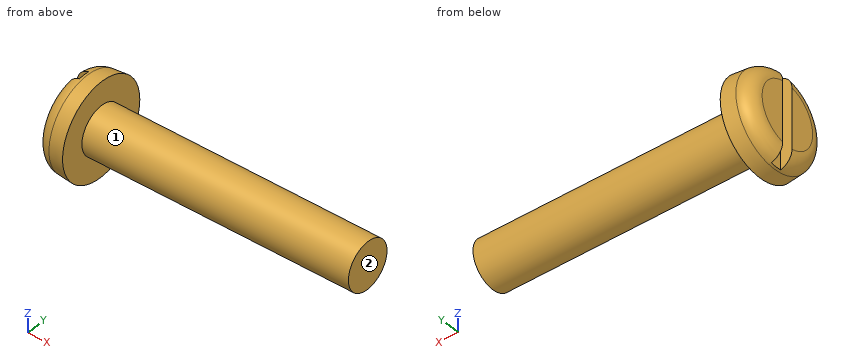
from build123d import *

# Parameters (mm, degrees)
FILLET2_R  = 0.8
SKETCH2_W  = 5
SKETCH2_H  = 0.6
SLOT_DEPTH = 0.6


with BuildPart() as part:
    # BodySke → Base-Revolve (revolve)
    with BuildSketch(Plane.XY):
        Polygon((1.5, 1.25), (1.5, 2.5), (0, 2.368767005), (0, 0), (15.5, 0), (15.5, 1.25), align=None)
    revolve(axis=Axis((-25.4, 0, 0), (1, 0, 0)))

    # Fillet2
    fillet2_edges = [part.edges().sort_by_distance(p)[0] for p in [
        (0, -2.368767005, 0),
    ]]
    fillet(fillet2_edges, radius=FILLET2_R)

    # Sketch2 → Slot (cut)
    with BuildSketch(Plane(origin=(0, 0, 0), x_dir=(0, 0, -1), z_dir=(1, 0, 0))):
        Rectangle(SKETCH2_W, SKETCH2_H)
    extrude(amount=SLOT_DEPTH, mode=Mode.SUBTRACT)


solid = part.part
Read the model definition and answer for the solid it produces. Units are mm, in the model's axes. Face numbers are marked on the shaded views. A direction names the side the tool comes from. Round coordinates to 2 decimals unless told otherwise and drop trailing zeros. Write each loop counter-clockwise with the first axis right and the second up, starting at its lowest first coordinate (ties: lowest second). Pieces come first, ordered by that corner, then holes.
1. The part is cut by section A-A, the plane y = 0. Determine the outline of the cut face in (x, z).
2. Which of the six approach directions +Z, -Z, +X, -X, +Y, -Y give full straight-line access (tool end or side, diameter ignored) to the marked faces 1 and 2?
3. Given pin 1 Ø2 at (x, z) = (13.5, -2) entering from +Y; pin 2 Ø2 at (x, y) = (6.5, -2) entering from -Z; pin 3 Ø0.5 at (x, z) = (0.5, 0) entering from -Y, each flat-ended and moving along its own axis, determine where each tip first touches the part or whether it passes through.
4. Straight lines are drawn through the part: L1, parallel to X at y = 1.2, z = -0.65; L2, parallel to X at y = -0.2, z = -0.1; L3, parallel to Z at x = 14, y = 0.05. For each, find the intervals that lie inside material, in ascending order.
5. The part is cut by section B-B, the plane z = 0. Determine the outline of the cut face in (x, y).
6. The part is cut by section C-C, the plane x = 14.5. Determine the outline of the cut face in (y, z), then the cut area to 3 significant figures.
Values:
1. outline: (0.6, -2.41) arc R0.8 ccw to (0.73, -2.43) - (1.5, -2.5) - (1.5, -1.25) - (15.5, -1.25) - (15.5, 1.25) - (1.5, 1.25) - (1.5, 2.5) - (0.73, 2.43) arc R0.8 ccw to (0.6, 2.41) - close
2. face 1: +X
2. face 2: +Z, -Z, +X, +Y, -Y
3. pin 1: stops at y = 0.75
3. pin 2: stops at z = -0.75
3. pin 3: stops at y = -2.43
4. L1: x = 0 to 1.5
4. L2: x = 0.6 to 15.5
4. L3: z = -1.25 to 1.25
5. outline: (0, -1.64) arc R0.8 ccw to (0.73, -2.43) - (1.5, -2.5) - (1.5, -1.25) - (15.5, -1.25) - (15.5, 1.25) - (1.5, 1.25) - (1.5, 2.5) - (0.73, 2.43) arc R0.8 ccw to (0, 1.64) - (0, 0.3) - (0.6, 0.3) - (0.6, -0.3) - (0, -0.3) - close
6. outline: circle Ø2.5 at (0, 0)
6. area: 4.91 mm2
